Work out the finished part from the listing and answer in its coordinate system (mm). Face numbers are marked on the shaded views. A direction names the side the tool comes from. Round coordinates to 2 decimals unless told otherwise and drop trailing zeros. Loops run counter-clockwise (first coordinate to the right, second up) from the corner with the lowest first, then second, coordinate; pieces in that order, holes last.
Autodesk Inventor part; units mm, degrees
ref_plane "YZ Plane" through (0, 0, 0) normal (1, 0, 0) x (0, 1, 0)
ref_plane "XZ Plane" through (0, 0, 0) normal (0, 1, 0) x (-1, 0, 0)
ref_plane "XY Plane" through (0, 0, 0) normal (0, 0, 1) x (1, 0, 0)
sketch "Sketch1" plane through (0, 0, 0) normal (0, 0, 1) x (1, 0, 0)
  line L0 (0, 0) -> (1270, 0)
  line L1 (1270, 0) -> (1270, 762)
  line L2 (1270, 762) -> (0, 762)
  line L3 (0, 762) -> (0, 0)
  dimension "d0" = 762
  dimension "d1" = 1270
extrude "Extrusion1" add sketch "Sketch1" along normal blind 127
sketch "Sketch2" plane through (0, 0, 127) normal (0, 0, 1) x (1, 0, 0)
  circle A0 centre (381, 381.7881) radius 76.2
  circle A1 centre (634.2119, 127) radius 76.2
  circle A2 centre (889, 380.2119) radius 76.2
  line L0 (0, 0) -> (1270, 0)
  line L1 (787.4, 394.1819) -> (990.6, 394.1819)
  line L2 (990.6, 394.1819) -> (990.6, 366.2419)
  line L3 (990.6, 366.2419) -> (787.4, 366.2419)
  line L4 (787.4, 366.2419) -> (787.4, 394.1819)
  line L5 (787.4, 394.1819) -> (990.6, 366.2419) construction
  line L6 (990.6, 394.1819) -> (787.4, 366.2419) construction
  line L7 (279.4, 395.7581) -> (482.6, 395.7581)
  line L8 (482.6, 395.7581) -> (482.6, 367.8181)
  line L9 (482.6, 367.8181) -> (279.4, 367.8181)
  line L10 (279.4, 367.8181) -> (279.4, 395.7581)
  line L11 (279.4, 395.7581) -> (482.6, 367.8181) construction
  line L12 (482.6, 395.7581) -> (279.4, 367.8181) construction
  line L13 (532.6119, 140.97) -> (735.8119, 140.97)
  line L14 (735.8119, 140.97) -> (735.8119, 113.03)
  line L15 (735.8119, 113.03) -> (532.6119, 113.03)
  line L16 (532.6119, 113.03) -> (532.6119, 140.97)
  line L17 (532.6119, 140.97) -> (735.8119, 113.03) construction
  line L18 (735.8119, 140.97) -> (532.6119, 113.03) construction
  point P0 (635, 381)
  point P1 (635, 0)
  point P2 (635, 0)
  point P3 (889, 380.2119)
  point P4 (381, 381.7881)
  point P5 (634.2119, 127)
  point P6 (306.0915, 367.8181)
  point P7 (306.0915, 395.7581)
  point P8 (455.9085, 395.7581)
  point P9 (455.9085, 367.8181)
  point P10 (709.1204, 140.97)
  point P11 (709.1204, 113.03)
  point P12 (559.3034, 113.03)
  point P13 (559.3034, 140.97)
  point P14 (963.9085, 394.1819)
  point P15 (963.9085, 366.2419)
  point P16 (814.0915, 366.2419)
  point P17 (814.0915, 394.1819)
  dimension "d14" = 152.4
  dimension "d17" = 180
  dimension "d19" = 127
  dimension "d20" = 381
  dimension "d23" = 203.2
  dimension "d24" = 27.94
  dimension "d25" = 203.2
  dimension "d26" = 27.94
  dimension "d27" = 203.2
  dimension "d28" = 27.94
extrude "Extrusion2" cut sketch "Sketch2" against normal blind 101.6
sketch "Sketch4" plane through (0, 0, 127) normal (0, 0, 1) x (1, 0, 0)
  line L0 (685.0119, 704.85) -> (939.0119, 704.85)
  line L1 (939.0119, 704.85) -> (939.0119, 615.95)
  line L2 (939.0119, 615.95) -> (685.0119, 615.95)
  line L3 (685.0119, 615.95) -> (685.0119, 704.85)
  line L4 (685.0119, 704.85) -> (939.0119, 615.95) construction
  line L5 (939.0119, 704.85) -> (685.0119, 615.95) construction
  line L6 (787.4, 394.1819) -> (814.0915, 394.1819)
  arc A0 (963.9085, 394.1819) -> (814.0915, 394.1819) centre (889, 380.2119) ccw
  line L7 (963.9085, 394.1819) -> (990.6, 394.1819)
  line L8 (990.6, 394.1819) -> (990.6, 366.2419)
  line L9 (990.6, 366.2419) -> (963.9085, 366.2419)
  arc A1 (814.0915, 366.2419) -> (963.9085, 366.2419) centre (889, 380.2119) ccw
  line L10 (814.0915, 366.2419) -> (787.4, 366.2419)
  line L11 (787.4, 366.2419) -> (787.4, 394.1819)
  line L12 (532.6119, 140.97) -> (559.3034, 140.97)
  arc A2 (709.1204, 140.97) -> (559.3034, 140.97) centre (634.2119, 127) ccw
  line L13 (709.1204, 140.97) -> (735.8119, 140.97)
  line L14 (735.8119, 140.97) -> (735.8119, 113.03)
  line L15 (735.8119, 113.03) -> (709.1204, 113.03)
  arc A3 (559.3034, 113.03) -> (709.1204, 113.03) centre (634.2119, 127) ccw
  line L16 (559.3034, 113.03) -> (532.6119, 113.03)
  line L17 (532.6119, 113.03) -> (532.6119, 140.97)
  line L18 (482.6, 367.8181) -> (455.9085, 367.8181)
  arc A4 (306.0915, 367.8181) -> (455.9085, 367.8181) centre (381, 381.7881) ccw
  line L19 (306.0915, 367.8181) -> (279.4, 367.8181)
  line L20 (279.4, 367.8181) -> (279.4, 395.7581)
  line L21 (279.4, 395.7581) -> (306.0915, 395.7581)
  arc A5 (455.9085, 395.7581) -> (306.0915, 395.7581) centre (381, 381.7881) ccw
  line L22 (455.9085, 395.7581) -> (482.6, 395.7581)
  line L23 (482.6, 395.7581) -> (482.6, 367.8181)
  line L24 (1270, 0) -> (1270, 762)
  line L25 (1270, 762) -> (0, 762)
  line L26 (0, 762) -> (0, 0)
  line L27 (0, 0) -> (1270, 0)
  line L28 (532.6119, 140.97) -> (532.6119, 113.03)
  line L29 (532.6119, 113.03) -> (559.3034, 113.03)
  arc A6 (559.3034, 113.03) -> (709.1204, 113.03) centre (634.2119, 127) ccw
  line L30 (709.1204, 113.03) -> (735.8119, 113.03)
  line L31 (735.8119, 113.03) -> (735.8119, 140.97)
  line L32 (735.8119, 140.97) -> (709.1204, 140.97)
  arc A7 (709.1204, 140.97) -> (559.3034, 140.97) centre (634.2119, 127) ccw
  line L33 (559.3034, 140.97) -> (532.6119, 140.97)
  line L34 (329.4119, 704.85) -> (583.4119, 704.85)
  line L35 (583.4119, 704.85) -> (583.4119, 615.95)
  line L36 (583.4119, 615.95) -> (329.4119, 615.95)
  line L37 (329.4119, 615.95) -> (329.4119, 704.85)
  line L38 (329.4119, 704.85) -> (583.4119, 615.95) construction
  line L39 (583.4119, 704.85) -> (329.4119, 615.95) construction
  line L40 (583.4119, 330.9881) -> (685.0119, 330.9881)
  line L41 (685.0119, 330.9881) -> (685.0119, 432.5881)
  line L42 (685.0119, 432.5881) -> (583.4119, 432.5881)
  line L43 (583.4119, 432.5881) -> (583.4119, 330.9881)
  line L44 (583.4119, 330.9881) -> (685.0119, 432.5881) construction
  line L45 (685.0119, 330.9881) -> (583.4119, 432.5881) construction
  point P0 (812.0119, 660.4)
  point P1 (634.2119, 653.1699)
  point P2 (456.4119, 660.4)
  point P3 (634.2119, 381.7881)
  dimension "d29" = 254
  dimension "d30" = 88.9
  dimension "d31" = 177.8
  dimension "d32" = 101.6
  dimension "d33" = 254
  dimension "d34" = 88.9
  dimension "d35" = 177.8
  dimension "d36" = 101.6
  dimension "d37" = 101.6
  dimension "d38" = 101.6
extrude "Extrusion3" add sketch "Sketch4" along normal blind 25.4 contours L0 L1 L2 L3 | L34 L35 L36 L37 | L43 L42 L41 L40
properties part number "Deska" material "Wood (Oak)"
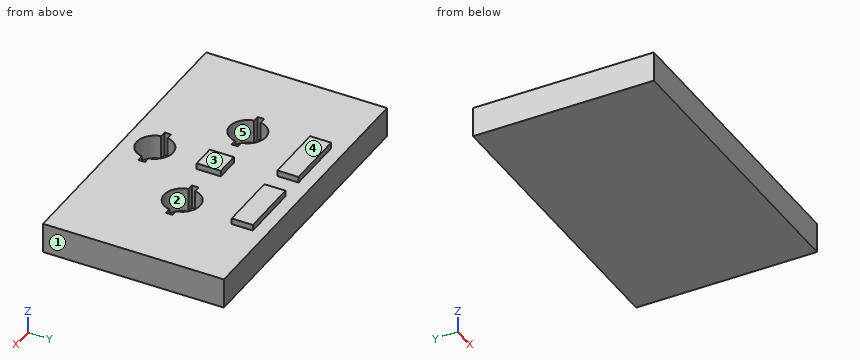
1. Given pin 1 (12.5 mm diameter, centred on x = 638.5, z = 143.5, fed in from -Y); pin 2 (21.5 mm diameter, centred on x = 543, z = 95, fed in from -Y); pin 3 (7.5 mm diameter, centred on y = 677.5, z = 142, fed in from +X); pin 4 (8 mm diameter, centred on x = 383.5, y = 170, fed in from +Z), each flat-ended and moving along its own axis, determine where each tip first touches the part or whether it passes through.
Answer key:
pin 1: stops at y = 330.99
pin 2: stops at y = 0
pin 3: stops at x = 939.01
pin 4: stops at z = 127
2. Consider probe 1 along X at (y, z) = (392, 79); probe 2 along X at (y, z) = (126.5, 116.5); probe 3 along X at (y, z) = (324, 29.5). Determine where each line is inside the solid, lowest interval first.
Answer key:
probe 1: x = 0 to 279.4, 482.6 to 787.4, 990.6 to 1270
probe 2: x = 0 to 532.61, 735.81 to 1270
probe 3: x = 0 to 331.33, 430.67 to 837.55, 940.45 to 1270
3. Find section D-D (x = 1006). Write down the section's boundary in (y, z), then the cut area to 3 significant figures.
Answer key:
outline: (0, 0) - (762, 0) - (762, 127) - (0, 127) - close
area: 96,800 mm2
4. Find section B-B (y = 634). Write down the section's boundary in (x, z).
Answer key:
outline: (0, 0) - (1270, 0) - (1270, 127) - (939.01, 127) - (939.01, 152.4) - (685.01, 152.4) - (685.01, 127) - (583.41, 127) - (583.41, 152.4) - (329.41, 152.4) - (329.41, 127) - (0, 127) - close
5. Find section A-A (z = 51.5). Write down the section's boundary in (x, y), then the cut area to 3 significant figures.
Answer key:
outline: (0, 0) - (1270, 0) - (1270, 762) - (0, 762) - close; hole (279.4, 367.82) - (306.09, 367.82) arc R76.2 ccw to (455.91, 367.82) - (482.6, 367.82) - (482.6, 395.76) - (455.91, 395.76) arc R76.2 ccw to (306.09, 395.76) - (279.4, 395.76) - close; hole (532.61, 113.03) - (559.3, 113.03) arc R76.2 ccw to (709.12, 113.03) - (735.81, 113.03) - (735.81, 140.97) - (709.12, 140.97) arc R76.2 ccw to (559.3, 140.97) - (532.61, 140.97) - close; hole (787.4, 366.24) - (814.09, 366.24) arc R76.2 ccw to (963.91, 366.24) - (990.6, 366.24) - (990.6, 394.18) - (963.91, 394.18) arc R76.2 ccw to (814.09, 394.18) - (787.4, 394.18) - close
area: 909,000 mm2
6. Which of the six approach directions +Z, -Z, +X, -X, +Y, -Y give full straight-line access (tool end or side, diameter ignored) to the marked faces 4 and 5?
Answer key:
face 4: +Z, +X, -X, +Y, -Y
face 5: +Z
7. Determine the mould class of the marked faces 1, 2 and 3 for opening direction X: +X half, -X half, draft (parallel to the pull), parting line (faces both ways), or undercut.
Answer key:
face 1: +X half
face 2: undercut
face 3: draft
8. Find section C-C (x = 751). Write down the section's boundary in (y, z).
Answer key:
outline: (0, 0) - (762, 0) - (762, 127) - (704.85, 127) - (704.85, 152.4) - (615.95, 152.4) - (615.95, 127) - (0, 127) - close
